```python
from build123d import *

# Parameters (mm, degrees)
BOSS_EXTRUDE1_DEPTH = 40
FILLET1_R           = 2


with BuildPart() as part:
    # Sketch1 → Boss-Extrude1 (new body)
    with BuildSketch(Plane(origin=(0, 0, 0), x_dir=(1, 0, 0), z_dir=(0, 1, 0))):
        Polygon((0, 0), (-2, 0), (-2, 6), (4, 6), (4, 4), (0, 4), (0, 0.889632107), align=None)
    extrude(amount=BOSS_EXTRUDE1_DEPTH)

    # Fillet1
    fillet1_edges = [part.edges().sort_by_distance(p)[0] for p in [
        (-2, 20, -6),
    ]]
    fillet(fillet1_edges, radius=FILLET1_R)


solid = part.part
```
The listing builds one solid part. Answer for the finished solid, in the listing's coordinates (mm). A direction names the side the tool comes from. Coordinates: 2 decimals unless noted, no trailing zeros. Write each loop counter-clockwise with the first axis right and the second up, starting at its lowest first coordinate (ties: lowest second). Pieces come first, ordered by that corner, then holes. Notation, with made-up numbers: (-10.5, 54) - (41.5, 54) arc R25 cw to (41.5, 91) - close; hole circle Ø1 at (35.25, 65.5). An arc over 180 degrees is marked (long way). Return JSON: item names as keys, results as strings. Group by question number.
Q1. The part is cut by section A-A on y = 22. Write down the section's boundary in (x, z).
Q2. Find the intervals of material crossed by line 1 along X through (y, z) = (5, -1.45); line 2 along Z through (x, y) = (0.65, 11); line 3 along Z through (x, y) = (-0.15, 18), in increasing order. Write a range as [from, to].
Q3. The part is cut by section C-C on x = 0.7. Write down the section's boundary in (y, z).
Q4. The part is cut by section B-B on z = -3.15. Write down the section's boundary in (x, y), and give its area (3 significant figures).
Q5. Which of the six approach directions +Z, -Z, +X, -X, +Y, -Y give full straight-line access (tool end or side, diameter ignored) to faces 1 (the flat face through (2, 20, -6)), 2 (the flat face through (0, 20, -2))?
Q6. Flat-ended cylindrical pins translate along their axes: pin 1 Ø2 at (y, z) = (14.5, -1.5) entering from +X; pin 2 Ø2 at (x, y) = (2.5, 27.5) entering from +Z. Find the tip coordinate at first contact, or state that the pin passes through.
Evaluation:
{
 "1": {"outline": "(-2, -4) arc R2 ccw to (0, -6) - (4, -6) - (4, -4) - (0, -4) - (0, 0) - (-2, 0) - close"},
 "2": {"line 1": "x = [-2, 0]", "line 2": "z = [-6, -4]", "line 3": "z = [-5.99, 0]"},
 "3": {"outline": "(0, -6) - (40, -6) - (40, -4) - (0, -4) - close"},
 "4": {"outline": "(-2, 0) - (0, 0) - (0, 40) - (-2, 40) - close", "area": "80.0 mm2"},
 "5": {"face 1": "-Z, +X, -X, +Y, -Y", "face 2": "+Z, +X, +Y, -Y"},
 "6": {"pin 1": "stops at x = 0", "pin 2": "stops at z = -4"}
}
